Model file for the job. Use its own axes, mm. Face numbers are marked on the shaded views. Give positions to 0.01 mm unless a question says otherwise; leave off trailing zeros. Write each loop counter-clockwise with the first axis right and the second up, starting at its lowest first coordinate (ties: lowest second). Pieces come first, ordered by that corner, then holes.
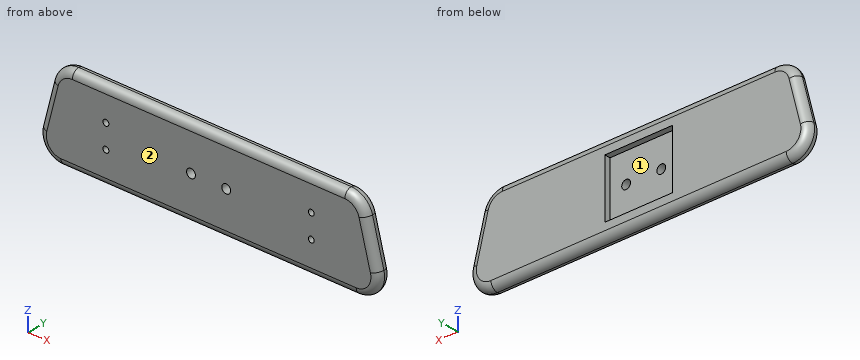
```python
from build123d import *

# Parameters (mm, degrees)
BOSS_EXTRUDE1_DEPTH = 10
SKETCH2_W           = 46
SKETCH2_H           = 40
CUT_EXTRUDE1_DEPTH  = 4
SKETCH2_3_R         = 3
CUT_EXTRUDE2_DEPTH  = 120.873502812
FILLET1_R           = 5
SKETCH3_R           = 2
CUT_EXTRUDE3_DEPTH  = 8


with BuildPart() as part:
    # Sketch1 → Boss-Extrude1 (new body)
    with BuildSketch(Plane(origin=(0, 0, 0), x_dir=(1, 0, 0), z_dir=(0, 1, 0))):
        with BuildLine():
            Line((115.149446157, 11.244299939), (107.390918627, -18.755700061))
            ThreePointArc((107.390918627, -18.755700061), (102.051963222, -26.860343606), (92.868704021, -30))
            Line((92.868704021, -30), (-92.868704021, -30))
            ThreePointArc((-92.868704021, -30), (-102.051963222, -26.860343606), (-107.390918627, -18.755700061))
            Line((-107.390918627, -18.755700061), (-115.149446157, 11.244299939))
            ThreePointArc((-115.149446157, 11.244299939), (-112.487575158, 24.183259201), (-100.627231552, 30))
            Line((-100.627231552, 30), (100.627231552, 30))
            ThreePointArc((100.627231552, 30), (112.487575158, 24.183259201), (115.149446157, 11.244299939))
        make_face()
    extrude(amount=BOSS_EXTRUDE1_DEPTH)

    # Sketch2 → Cut-Extrude1 (cut)
    with BuildSketch(Plane(origin=(0, 10, 0), x_dir=(1, 0, 0), z_dir=(0, 1, 0))):
        Rectangle(SKETCH2_W, SKETCH2_H)
    extrude(amount=-CUT_EXTRUDE1_DEPTH, mode=Mode.SUBTRACT)

    # Sketch2<3> → Cut-Extrude2 (cut, through all)
    with BuildSketch(Plane(origin=(0, 10, 0), x_dir=(1, 0, 0), z_dir=(0, 1, 0))):
        with Locations(Location((-12, 0, 0), (0, 0, 270))):
            Circle(SKETCH2_3_R)
        with Locations(Location((12, 0, 0), (0, 0, 270))):
            Circle(SKETCH2_3_R)
    extrude(amount=-CUT_EXTRUDE2_DEPTH, mode=Mode.SUBTRACT)

    # Fillet1
    fillet1_edges = [part.edges().sort_by_distance(p)[0] for p in [
        (0, 0, 30),
        (-102.051963222, 0, 26.860343606),
        (-111.270182392, 0, 3.755700061),
        (-112.487575158, 0, -24.183259201),
        (0, 10, 30),
        (102.051963222, 10, 26.860343606),
        (111.270182392, 10, 3.755700061),
        (112.487575158, 10, -24.183259201),
        (0, 10, -30),
        (0, 0, -30),
        (-111.270182392, 10, 3.755700061),
        (111.270182392, 0, 3.755700061),
    ]]
    fillet(fillet1_edges, radius=FILLET1_R - 0.0001)  # a hair under: the kernel refuses the full size

    # Sketch3 → Cut-Extrude3 (cut)
    with BuildSketch(Plane.XZ):
        with Locations(Location((-70, 8, 0), (0, 0, 270))):
            Circle(SKETCH3_R)
        with Locations(Location((-70, -8, 0), (0, 0, 90))):
            Circle(SKETCH3_R)
        with Locations(Location((70, -8, 0), (0, 0, 270))):
            Circle(SKETCH3_R)
        with Locations(Location((70, 8, 0), (0, 0, 90))):
            Circle(SKETCH3_R)
    extrude(amount=-CUT_EXTRUDE3_DEPTH, mode=Mode.SUBTRACT)


solid = part.part
```
1. Probe probe 1 along X at (y, z) = (2, -8); probe 2 along X at (y, z) = (2.1, 0); probe 3 along X at (y, z) = (2.5, 16). List the from-to ranges inside material, lowest first.
Calculated:
probe 1: x = -113.28 to -72, -68 to 68, 72 to 113.28
probe 2: x = -111.28 to -15, -9 to 9, 15 to 111.28
probe 3: x = -107.41 to 107.41
2. Pin check, flat tips, straight feed: P1, Ø1.5, axis at y = 7, z = -7, coming from the +X side; P2, Ø4.5, axis at y = 8.5, z = -5, coming from the +X side; P3, Ø2, axis at y = 7.5, z = -2.5, coming from the -X side; P4, Ø5, axis at x = -12, z = 0, coming from the -Y side. Stop position of each tip, or through.
Calculated:
P1: stops at x = 113.96
P2: stops at x = 113.58
P3: stops at x = -112.74
P4: passes through
3. Slice it at C-C, the plane y = 2.75. Write the cut outline in (x, z), and give its area (3 significant figures).
Calculated:
outline: (-114.63, -11.38) arc R14.47 ccw to (-100.63, -29.47) - (100.63, -29.47) arc R14.47 ccw to (114.63, -11.38) - (106.87, 18.62) arc R14.47 ccw to (92.87, 29.47) - (-92.87, 29.47) arc R14.47 ccw to (-106.87, 18.62) - close; hole circle Ø4 at (-70, -8); hole circle Ø4 at (-70, 8); hole circle Ø6 at (-12, 0); hole circle Ø6 at (12, 0); hole circle Ø4 at (70, -8); hole circle Ø4 at (70, 8)
area: 12,800 mm2
4. Pull direction Z, two halves, no side cores. Call the marked faces 1 and 2: +Z half, -Z half, draft (parallel to the pull), parting line (faces both ways), or undercut.
Calculated:
face 1: undercut
face 2: draft
